Design review of the part built by this model. Coordinates are the model's own, in mm. Coordinates: 2 decimals unless noted, no trailing zeros. Loops run counter-clockwise (first coordinate to the right, second up) from the corner with the lowest first, then second, coordinate; pieces in that order, holes last. Notation, with made-up numbers: M -35.5,-5.5 L 21.5,-5.5 A22 cw 21.5,17.5 Z; hole C 30.25,10 d11. An arc over 180 degrees is marked long. Put each result on its own line as item: value. Start each with the question number.
(1) Take a section at B-B, the plane z = 0.5. Give the boundary of the cut face in (x, y).
(2) Take a section at A-A, the plane x = 0. Give the boundary of the cut face in (y, z), then the cut area to 3 significant figures.
(3) Clearance check with flat-ended pins moving along their axes: pin 1 (2.5 mm diameter, centred on x = 8.78, z = -9.09, fed in from -Y); pin 2 (1.4 mm diameter, centred on x = -13, y = -1.5, fed in from +Z). State where each tip first meets the part, or that it passes through.
(4) Take a section at C-C, the plane z = -7. Give the boundary of the cut face in (x, y).
(5) Take a section at D-D, the plane y = -0.5. Count the separate pieces of the cut face and the enclosed holes in it, then the cut area to 3 significant figures.
(6) For probe 1 along X at (y, z) = (-1.85, 0.5); probe 2 along Z at (x, y) = (1.5, -2.5); probe 3 along X at (y, z) = (-1.25, -0.75), list the stretches that pass through material, from the lowest coordinate up. Write a range as [from, to].
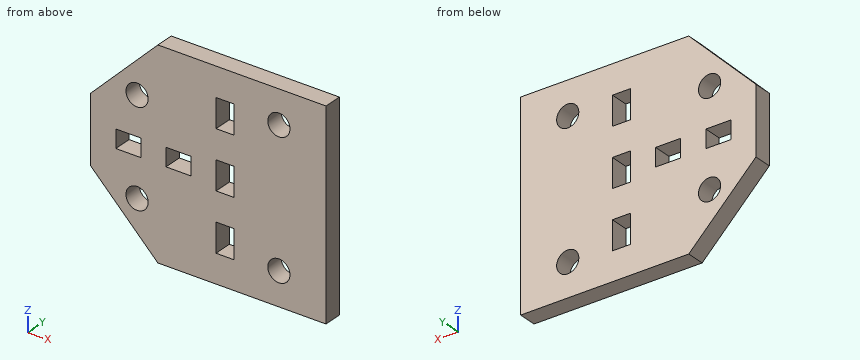
```python
from build123d import *

# Parameters (mm, degrees)
SKETCH1_R           = 1.65
SKETCH1_W           = 2.7
SKETCH1_H           = 4.285714286
SKETCH1_H_2         = 4.285714285
SKETCH1_W_2         = 3.73
SKETCH1_H_3         = 2.7
BOSS_EXTRUDE1_DEPTH = 2.7


with BuildPart() as part:
    # Sketch1 → Boss-Extrude1 (new body)
    with BuildSketch(Plane(origin=(0, 0, 0), x_dir=(1, 0, 0), z_dir=(0, 1, 0))):
        Polygon((10.776704041, -15.946127132), (-9.223295959, -15.946127132), (-19.223295959, -5.946127132), (-19.223295959, 4.053872868), (-9.223295959, 14.053872868), (10.776704041, 14.053872868), (15.776704041, 14.053872868), (15.776704041, -15.946127132), align=None)
        with Locations((-12.32618077, -8.023001304)):
            Circle(SKETCH1_R, mode=Mode.SUBTRACT)
        with Locations((8.776704041, 9.093845285)):
            Circle(SKETCH1_R, mode=Mode.SUBTRACT)
        with Locations((-12.32618077, 6.210691875)):
            Circle(SKETCH1_R, mode=Mode.SUBTRACT)
        with Locations((8.776704041, -10.98609955)):
            Circle(SKETCH1_R, mode=Mode.SUBTRACT)
        with Locations((0.776704041, -9.477583286)):
            Rectangle(SKETCH1_W, SKETCH1_H, mode=Mode.SUBTRACT)
        with Locations((0.776704041, -0.906154715)):
            Rectangle(SKETCH1_W, SKETCH1_H, mode=Mode.SUBTRACT)
        with Locations((0.776704041, 7.665273857)):
            Rectangle(SKETCH1_W, SKETCH1_H_2, mode=Mode.SUBTRACT)
        with Locations((-13.628295959, -0.938132649)):
            Rectangle(SKETCH1_W_2, SKETCH1_H_3, mode=Mode.SUBTRACT)
        with Locations((-6.168295959, -0.922143682)):
            Rectangle(SKETCH1_W_2, SKETCH1_H_3, mode=Mode.SUBTRACT)
    extrude(amount=-BOSS_EXTRUDE1_DEPTH)


solid = part.part
```
Computed values:
1. outline: M -19.22,-2.7 L -15.49,-2.7 L -15.49,0 L -19.22,0 Z; M -11.76,-2.7 L -8.03,-2.7 L -8.03,0 L -11.76,0 Z; M -4.3,-2.7 L -0.57,-2.7 L -0.57,0 L -4.3,0 Z; M 2.13,-2.7 L 15.78,-2.7 L 15.78,0 L 2.13,0 Z
2. outline: M -2.7,-14.05 L 0,-14.05 L 0,-9.81 L -2.7,-9.81 Z; M -2.7,-5.52 L 0,-5.52 L 0,-1.24 L -2.7,-1.24 Z; M -2.7,3.05 L 0,3.05 L 0,7.33 L -2.7,7.33 Z; M -2.7,11.62 L 0,11.62 L 0,15.95 L -2.7,15.95 Z
2. area: 46.3 mm^2
3. pin 1: passes through
3. pin 2: stops at z = 12.87
4. outline: M -16.28,-2.7 L -13.78,-2.7 L -13.78,0 L -16.28,0 Z; M -10.88,-2.7 L -0.57,-2.7 L -0.57,0 L -10.88,0 Z; M 2.13,-2.7 L 15.78,-2.7 L 15.78,0 L 2.13,0 Z
5. separate pieces: 1
5. enclosed holes: 9
5. area: 861 mm^2
6. probe 1: x = [-19.22, -15.49], [-11.76, -8.03], [-4.3, -0.57], [2.13, 15.78]
6. probe 2: z = [-14.05, -9.81], [-5.52, -1.24], [3.05, 7.33], [11.62, 15.95]
6. probe 3: x = [-19.22, -0.57], [2.13, 15.78]
